```python
from build123d import *

# Parameters (mm, degrees)
F0_W     = 58.9296072721
F0_H     = 55.0467334688
F1_DEPTH = 25.4
F3_DEPTH = 34.68607


with BuildPart() as f1:
    # F0 (on Top) → F1 (new body)
    with BuildSketch(Plane.XY):
        with Locations((-29.4648036361, 3.4594554454)):
            Rectangle(F0_W, F0_H)
    extrude(amount=F1_DEPTH)

    # F2 (on face) → F3 (cut)
    with BuildSketch(Plane.XY.offset(25.4)):
        with BuildLine():
            ThreePointArc((-52.1536211312, 8.0381335624), (-35.3203383975, 5.3039070161), (-26.0133259195, 19.5942856371))
            ThreePointArc((-26.0133259195, 19.5942856371), (-27.29800697, 25.7986930506), (-30.9407918835, 30.9828221798))
            Line((-30.9407918835, 30.9828221798), (-34.4491236613, 30.9828221798))
            ThreePointArc((-34.4491236613, 30.9828221798), (-44.147413461, 20.163297011), (-52.1536211312, 8.0381335624))
        make_face()
        with BuildLine():
            ThreePointArc((-52.334921143, 30.9828221798), (-57.2618993675, 19.470830523), (-52.1536211312, 8.0381335624))
            ThreePointArc((-52.1536211312, 8.0381335624), (-44.147413461, 20.163297011), (-34.4491236613, 30.9828221798))
            Line((-34.4491236613, 30.9828221798), (-52.334921143, 30.9828221798))
        make_face()
        with BuildLine():
            ThreePointArc((-34.4491236613, 30.9828221798), (-33.6460547954, 31.7472714752), (-32.834456283, 32.5026589143))
            ThreePointArc((-32.834456283, 32.5026589143), (-42.8519269969, 35.1715764522), (-52.334921143, 30.9828221798))
            Line((-52.334921143, 30.9828221798), (-34.4491236613, 30.9828221798))
        make_face()
    extrude(amount=-F3_DEPTH, mode=Mode.SUBTRACT)


solid = f1.part
```
For this review, take the finished solid that the model builds, in its own axes (mm). Give positions to 0.01 mm unless a question says otherwise; leave off trailing zeros. Order: outer loops, then holes, each group sorted by start corner. A loop starts at its lowest first (then second) coordinate and runs counter-clockwise, first axis right, second up.
1) Take a section at A-A (z = 11.5). Give the boundary of the cut face in (x, y), then the cut area to 3 significant figures.
2) Wall thickness on line 1 (X direction, y = 29, z = 14.5); line 2 (X direction, y = 14, z = 23.5); line 3 (Y direction, x = -28.5, z = 6.5): over which ranges is each line inside the solid? List them lowest first.
3) Take a section at D-D (x = -33). Give the boundary of the cut face in (y, z), then the cut area to 3 significant figures.
4) Take a section at B-B (y = 13.5). Give the boundary of the cut face in (x, z).
5) Insertion check: pin 1 (12 mm diameter, centred on x = -27, y = 11, fed in from -Z). The pin has a flat end and moves straight along its axis. Give the tip position at first contact, or say it passes through.
6) Take a section at C-C (x = -43). Give the boundary of the cut face in (y, z), then the cut area to 3 significant figures.
Derived:
1. outline: (-58.93, -24.06) - (0, -24.06) - (0, 30.98) - (-30.94, 30.98) arc R15.62 cw (long way) to (-52.33, 30.98) - (-58.93, 30.98) - close
1. area: 2,540 mm2
2. line 1: x = -58.93 to -54.11, -29.16 to 0
2. line 2: x = -58.93 to -56.23, -27.05 to 0
2. line 3: y = -24.06 to 11.14, 28.05 to 30.98
3. outline: (-24.06, 0) - (6.57, 0) - (6.57, 25.4) - (-24.06, 25.4) - close
3. area: 778 mm2
4. outline: (-58.93, 0) - (-56.02, 0) - (-56.02, 25.4) - (-58.93, 25.4) - close; (-27.25, 0) - (0, 0) - (0, 25.4) - (-27.25, 25.4) - close
5. pin 1: stops at z = 0
6. outline: (-24.06, 0) - (4.03, 0) - (4.03, 25.4) - (-24.06, 25.4) - close
6. area: 714 mm2
